Could you check a few things on this model? Use its own coordinates, in mm. Face numbers are marked on the shaded views. A direction names the side the tool comes from. Coordinates: 2 decimals unless noted, no trailing zeros. Write each loop counter-clockwise with the first axis right and the second up, starting at its lowest first coordinate (ties: lowest second). Pieces come first, ordered by that corner, then holes. Notation, with made-up numbers: M 68.5,-11 L 117.5,-11 A28 cw 117.5,24 Z; hole C 24.25,56 d4. An arc over 180 degrees is marked long. Write item = value, one per line.
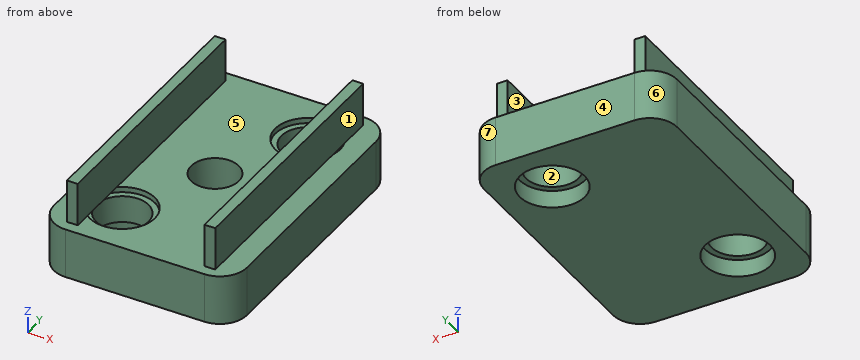
```python
from build123d import *

# Parameters (mm, degrees)
BOSS_EXTRUDE1_DEPTH = 4.6
SKETCH4_R           = 2.425
CUT_EXTRUDE1_DEPTH  = 14.6
SKETCH5_R           = 3
CUT_EXTRUDE2_DEPTH  = 1.6
SKETCH6_R           = 3
CUT_EXTRUDE3_DEPTH  = 0.5
SKETCH7_R           = 2.2
CUT_EXTRUDE4_DEPTH  = 3
SKETCH8_W           = 1
SKETCH8_H           = 23.79
BOSS_EXTRUDE2_DEPTH = 4


with BuildPart() as part:
    # Sketch1 → Boss-Extrude1 (new body)
    with BuildSketch(Plane.XY):
        with BuildLine():
            Line((2.5, 0), (15.32, 0))
            ThreePointArc((15.32, 0), (17.087766953, 0.732233047), (17.82, 2.5))
            Line((17.82, 2.5), (17.82, 23.29))
            ThreePointArc((17.82, 23.29), (17.087766953, 25.057766953), (15.32, 25.79))
            Line((15.32, 25.79), (2.5, 25.79))
            ThreePointArc((2.5, 25.79), (0.732233047, 25.057766953), (0, 23.29))
            Line((0, 23.29), (0, 2.5))
            ThreePointArc((0, 2.5), (0.732233047, 0.732233047), (2.5, 0))
        make_face()
    extrude(amount=BOSS_EXTRUDE1_DEPTH)

    # Sketch4 → Cut-Extrude1 (cut)
    with BuildSketch(Plane.XY.offset(4.6)):
        with Locations((4.925, 4.925)):
            Circle(SKETCH4_R)
        with Locations((12.895, 20.865)):
            Circle(SKETCH4_R)
    extrude(amount=-CUT_EXTRUDE1_DEPTH, mode=Mode.SUBTRACT)

    # Sketch5 → Cut-Extrude2 (cut)
    with BuildSketch(Plane(origin=(0, 0, 0), x_dir=(-1, 0, 0), z_dir=(0, 0, -1))):
        with Locations((-12.895, 20.865)):
            Circle(SKETCH5_R)
        with Locations((-4.925, 4.925)):
            Circle(SKETCH5_R)
    extrude(amount=-CUT_EXTRUDE2_DEPTH, mode=Mode.SUBTRACT)

    # Sketch6 → Cut-Extrude3 (cut)
    with BuildSketch(Plane.XY.offset(4.6)):
        with Locations((4.925, 4.925)):
            Circle(SKETCH6_R)
        with Locations((12.895, 20.865)):
            Circle(SKETCH6_R)
    extrude(amount=-CUT_EXTRUDE3_DEPTH, mode=Mode.SUBTRACT)

    # Sketch7 → Cut-Extrude4 (cut)
    with BuildSketch(Plane.XY.offset(4.6)):
        with Locations((8.91, 12.895)):
            Circle(SKETCH7_R)
    extrude(amount=-CUT_EXTRUDE4_DEPTH, mode=Mode.SUBTRACT)

    # Sketch8 → Boss-Extrude2 (add)
    with BuildSketch(Plane.XY.offset(4.6)):
        with Locations((2.56, 12.895)):
            Rectangle(SKETCH8_W, SKETCH8_H)
        with Locations((15.26, 12.895)):
            Rectangle(SKETCH8_W, SKETCH8_H)
    extrude(amount=BOSS_EXTRUDE2_DEPTH)


solid = part.part
```
Item 1: If we mould it in two halves opening along X, with no side actions, what happens to the marked faces 4, 5, 6 and 7? For each: pulls with the +X half, pulls with the -X half, needs draft (parallel to the pull), parting line crosses it, or undercut.
Numbers:
face_4 = needs draft
face_5 = undercut
face_6 = pulls with the -X half
face_7 = pulls with the +X half
Item 2: Imagine slicing it at D-D (x = 14.25). Write out the boundary of the cut face in (y, z).
Numbers:
outline = M 0,0 L 18.19,0 L 18.19,1.6 L 18.85,1.6 L 18.85,4.1 L 18.19,4.1 L 18.19,4.6 L 0,4.6 Z; M 22.88,1.6 L 23.54,1.6 L 23.54,0 L 25.79,0 L 25.79,4.6 L 23.54,4.6 L 23.54,4.1 L 22.88,4.1 Z
Item 3: Imagine slicing it at C-C (y = 8.25). Write out the boundary of the cut face in (x, z), and give its area (3 significant figures).
Numbers:
outline = M 0,0 L 17.82,0 L 17.82,4.6 L 15.76,4.6 L 15.76,8.6 L 14.76,8.6 L 14.76,4.6 L 3.06,4.6 L 3.06,8.6 L 2.06,8.6 L 2.06,4.6 L 0,4.6 Z
area = 90.0 mm²
Item 4: Imagine slicing it at A-A (z = 7). Write out the boundary of the cut face in (x, y).
Numbers:
outline = M 2.06,1 L 3.06,1 L 3.06,24.79 L 2.06,24.79 Z; M 14.76,1 L 15.76,1 L 15.76,24.79 L 14.76,24.79 Z
Item 5: For the marked faces 1, 2 and 3, which set-ups out of +Z, -Z, +X, -X, +Y, -Y let a thin tool reach every point of the face, with its end or its side?
Numbers:
face_1 = +Z, +X, +Y, -Y
face_2 = -Z
face_3 = +Z, +Y, -Y
Item 6: Imagine slicing it at B-B (x = 8.91). Write out the boundary of the cut face in (y, z) (3 decimals), and give its area (3 significant figures).
Numbers:
outline = M 0,0 L 25.79,0 L 25.79,4.6 L 15.095,4.6 L 15.095,1.6 L 10.695,1.6 L 10.695,4.6 L 0,4.6 Z
area = 105 mm²
Item 7: I'm going to push flat-ended pins straight in: P1, Ø5, axis at x = 4.925, y = 4.925, coming from the -Z side; P2, Ø0.8, axis at x = 2.5, z = 6.5, coming from the +Y side; P3, Ø6, axis at x = 10, y = 21.5, coming from the +Z side. Where does each tip first touch, or does it pass through?
Numbers:
P1 = 1.6
P2 = 24.79
P3 = 4.6
Item 8: If I drill on line 1 along Y through (x, z) = (5, 3); line 2 along X through (y, z) = (24.5, 6); line 3 along Y through (x, z) = (13, 3.25), over which ranges is the centre line in solid material (lowest first)?
Numbers:
line_1 = 0 to 2.5, 7.35 to 25.79
line_2 = 2.06 to 3.06, 14.76 to 15.76
line_3 = 0 to 18.44, 23.29 to 25.79
